```python
from build123d import *

# Parameters (mm, degrees)
SKETCH_1_W      = 120
SKETCH_1_H      = 147.25
EXTRUDE_1_DEPTH = 40
SKETCH_2_W      = 50.114502488
SKETCH_2_H      = 40
SKETCH_2_W_2    = 54.885497512
EXTRUDE_2_DEPTH = 12
SKETCH_3_R      = 24
SKETCH_3_R_2    = 12.5
EXTRUDE_3_DEPTH = 35
SKETCH_4_W      = 120
SKETCH_4_H      = 100
EXTRUDE_4_DEPTH = 10


with BuildPart() as part:
    # 草图1 → 凸台-拉伸1 (new body)
    with BuildSketch(Plane.XY):
        with Locations((2.385497512, -49.600771144)):
            Rectangle(SKETCH_1_W, SKETCH_1_H)
    extrude(amount=EXTRUDE_1_DEPTH)

    # 草图2 → 凸台-拉伸2 (add)
    with BuildSketch(Plane(origin=(0, 24.024228856, 0), x_dir=(1, 0, 0), z_dir=(0, 1, 0))):
        with Locations((-32.557251244, -20)):
            Rectangle(SKETCH_2_W, SKETCH_2_H)
        with Locations((34.942748756, -20)):
            Rectangle(SKETCH_2_W_2, SKETCH_2_H)
    extrude(amount=EXTRUDE_2_DEPTH)

    # 草图3 → 凸台-拉伸3 (add)
    with BuildSketch(Plane.XY.offset(40)):
        with Locations((0, -75.475771144)):
            Circle(SKETCH_3_R)
        with Locations((0, -75.475771144)):
            Circle(SKETCH_3_R_2, mode=Mode.SUBTRACT)
    extrude_3 = extrude(amount=EXTRUDE_3_DEPTH)

    # 镜向1: 凸台-拉伸3 across plane
    add(extrude_3.mirror(Plane.XY.offset(20)))

    # 草图4 → 凸台-拉伸4 (add)
    with BuildSketch(Plane.XZ.offset(123.225771144)):
        with Locations((2.385497512, 20)):
            Rectangle(SKETCH_4_W, SKETCH_4_H)
    extrude(amount=-EXTRUDE_4_DEPTH)


solid = part.part
```
Here's how the part is built. I have some questions about the finished solid (model axes, mm). A direction names the side the tool comes from. Round coordinates to 2 decimals unless told otherwise and drop trailing zeros. Write each loop counter-clockwise with the first axis right and the second up, starting at its lowest first coordinate (ties: lowest second). Pieces come first, ordered by that corner, then holes. Notation, with made-up numbers: M 71.25,73 L 117.25,73 A13 cw 117.25,85 Z; hole C 57,40.25 d4. An arc over 180 degrees is marked long. Answer as CSV lines item,"result". Start each with the question number.
1. On a 3-axis mill with a long thin cutter (end or side, diameter ignored), from which of +Z, -Z, +X, -X, +Y, -Y can I reach the whole of each face in a straight line? I mean faces 5 (the flat face through (0, 24.024, 20)), 6 (the flat face through (2, -118, -30)), 7 (the flat face through (0, -76, 40)), 8 (the flat face through (2, -113.226, -15)), 9 (the flat face through (0, -76, 0)). Say none if no direction works.
2. Thinking about a two-plate mould opening in X: for faces 1 (the cylindrical face through (-2.71, -87.68, -17.26)), 2 (the cylindrical face through (-5.203, -98.905, -17.255)), 3 (the flat face through (2, -113.226, 55)), 4 (the flat face through (7.5, 30, 20)), which applies, released by +X, released by -X, zero draft, split by the parting line, or undercut?
3. Suppose I cut it at A-A on x = 0. Write out the boundary of the cut face in (y, z).
4. I'm going to push flat-ended pins straight in: pin 1 Ø6 at (x, y) = (-24, -25.5) entering from -Z; pin 2 Ø15 at (x, y) = (0, -75.48) entering from +Z; pin 3 Ø4.5 at (x, z) = (2, 18) entering from +Y. Where does each tip first touch, or does it pass through?
5. Suppose I cut it at D-D on x = 54. Write out the boundary of the cut face in (y, z), then the cut area to 3 significant figures.
6. I need wall thicknesses on probe 1 along Y at (x, z) = (0, 47.5); probe 2 along Z at (x, y) = (4, -104); probe 3 along Y at (x, z) = (27, 55.5). Which ranges of each line are inside material? Lowest first, please.
7. Suppose I cut it at C-C on y = -72. Write out the boundary of the cut face in (x, z), then the cut area to 3 significant figures.
8. Suppose I cut it at B-B on z = 62. Write out the boundary of the cut face in (x, y).
Check result:
1,face 5,"+Z, -Z, +Y"
1,face 6,"-Z, +X, -X, -Y"
1,face 7,"+Z"
1,face 8,"-Z, +X, -X"
1,face 9,"-Z"
2,face 1,"undercut"
2,face 2,"split by the parting line"
2,face 3,"zero draft"
2,face 4,"undercut"
3,outline,"M -123.23,-30 L -113.23,-30 L -113.23,0 L -99.48,0 L -99.48,-35 L -87.98,-35 L -87.98,0 L -62.98,0 L -62.98,-35 L -51.48,-35 L -51.48,0 L 24.02,0 L 24.02,40 L -51.48,40 L -51.48,75 L -62.98,75 L -62.98,40 L -87.98,40 L -87.98,75 L -99.48,75 L -99.48,40 L -113.23,40 L -113.23,70 L -123.23,70 Z"
4,pin 1,"stops at z = 0"
4,pin 2,"stops at z = 40"
4,pin 3,"stops at y = 24.02"
5,outline,"M -123.23,-30 L -113.23,-30 L -113.23,0 L 36.02,0 L 36.02,40 L -113.23,40 L -113.23,70 L -123.23,70 Z"
5,area,"6,970 mm2"
6,probe 1,"y = -123.23 to -113.23, -99.48 to -87.98, -62.98 to -51.48"
6,probe 2,"z = 0 to 40"
6,probe 3,"y = -123.23 to -113.23"
7,outline,"M -57.61,0 L -23.75,0 L -23.75,-35 L -12.01,-35 L -12.01,0 L 12.01,0 L 12.01,-35 L 23.75,-35 L 23.75,0 L 62.39,0 L 62.39,40 L 23.75,40 L 23.75,75 L 12.01,75 L 12.01,40 L -12.01,40 L -12.01,75 L -23.75,75 L -23.75,40 L -57.61,40 Z"
7,area,"6,440 mm2"
8,outline,"M -57.61,-123.23 L 62.39,-123.23 L 62.39,-113.23 L -57.61,-113.23 Z; C 0,-75.48 d48; hole C 0,-75.48 d25"
